Geometry: final body of the model. Coordinates: model frame, mm. A direction names the side the tool comes from. Give positions to 0.01 mm unless a question says otherwise; leave off trailing zeros. Write each loop counter-clockwise with the first axis right and the second up, starting at its lowest first coordinate (ties: lowest second). Pieces come first, ordered by that corner, then holes. Notation, with made-up numbers: M 85,58.5 L 93,58.5 A23 ccw 93,96.5 Z; hole C -12.5,-0.75 d3. An arc over 180 degrees is marked long. Use a Markdown table: item, result. Add a question column.
1) Section C-C on y = 42. Return the cut outline in (x, z), then the cut area to 3 significant figures.
2) Section B-B on z = 33. Return the cut outline in (x, y).
3) Set-up query: faces 1 (the cylindrical face through (4.83, 4.93, 18.22)), 2 (the flat face through (5, 43, 34)), 3 (the cylindrical face through (7.62, 3.78, 2)), 4 (the cylindrical face through (4.763, 77.521, 18.835)), 5 (the flat face through (7.5, 77, 34)). Return all of +Z, -Z, +X, -X, +Y, -Y with unobstructed straight access to the full face (end or side cutting, diameter ignored); none if empty.
4) Line query: line 1 (Z direction, x = 3.5, y = 4.5); line 2 (Y direction, x = 0.5, z = 27.5); line 3 (Z direction, x = 5, y = 2.5). Output: solid intervals per line, ascending.
5) Pin query (flat end, axial travel): pin 1 (4 mm diameter, centred on x = 11.5, z = 30, fed in from +Y); pin 2 (5 mm diameter, centred on x = 5, z = 21.5, fed in from +Y); pin 3 (2.5 mm diameter, centred on y = 77.5, z = 33, fed in from +X); pin 4 (2.5 mm diameter, centred on y = 41, z = 2, fed in from +X). Return the tip coordinate at first contact, or that it passes through.
6) Section D-D on z = 23. Return the cut outline in (x, y).
7) Draft query along X for faces 6 (the flat face through (7.5, 77, 4)), 7 (the cylindrical face through (4.733, 66.033, 36.028)), 8 (the flat face through (3, 76, 18)). Return one class per face: +X half, -X half, draft (parallel to the pull), parting line (faces both ways), or undercut.
8) Section A-A on y = 64. Return the cut outline in (x, z), then the cut area to 3 significant figures.
```python
from build123d import *

# Parameters (mm, degrees)
PAD_DEPTH       = 38
SKETCH001_R     = 2.05
POCKET_DEPTH    = 17.363189
SKETCH002_W     = 66
SKETCH002_H     = 31
POCKET001_DEPTH = 15.241
SKETCH003_R     = 2.05
POCKET002_DEPTH = 38.001
SKETCH004_W     = 3
SKETCH004_H     = 38
POCKET003_DEPTH = 2.5
POCKET004_DEPTH = 5
SKETCH006_R     = 0.8
POCKET005_DEPTH = 15


with BuildPart() as part:
    # Sketch → Pad (new body)
    with BuildSketch(Plane.XY):
        Polygon((15, 0), (0, 0), (0, 79), (10, 79), (10, 10), (15.24, 8), align=None)
    extrude(amount=PAD_DEPTH)

    # Sketch001 (on Face6 of Pad) → Pocket (cut, through all)
    with BuildSketch(Plane(origin=(14.986512, -0.449595, 0), x_dir=(0.029987, 0.99955, 0), z_dir=(0.99955, -0.029987, 0))):
        with Locations((4.451597, 34)):
            Circle(SKETCH001_R)
        with Locations((4.451597, 4)):
            Circle(SKETCH001_R)
    extrude(amount=-POCKET_DEPTH, mode=Mode.SUBTRACT)

    # Sketch002 (on Face3 of Pocket) → Pocket001 (cut, through all)
    with BuildSketch(Plane(origin=(0, 0, 0), x_dir=(0, -1, 0), z_dir=(-1, 0, 0))):
        with Locations((-43, 18.5)):
            Rectangle(SKETCH002_W, SKETCH002_H)
    extrude(amount=-POCKET001_DEPTH, mode=Mode.SUBTRACT)

    # Sketch003 (on Face5 of Pocket001) → Pocket002 (cut, through all)
    with BuildSketch(Plane.XY.offset(38)):
        with Locations((5, 64)):
            Circle(SKETCH003_R)
    extrude(amount=-POCKET002_DEPTH, mode=Mode.SUBTRACT)

    # Sketch004 (on Face14 of Pocket002) → Pocket003 (cut)
    with BuildSketch(Plane.YZ.offset(10)):
        with Locations((77.5, 19)):
            Rectangle(SKETCH004_W, SKETCH004_H)
    extrude(amount=-POCKET003_DEPTH, mode=Mode.SUBTRACT)

    # Sketch005 (on Face9 of Pocket003) → Pocket004 (cut)
    with BuildSketch(Plane(origin=(0, 79, 0), x_dir=(-1, 0, 0), z_dir=(0, 1, 0))):
        with BuildLine():
            ThreePointArc((-7.5, 7.624688), (-4.762126, 19), (-7.5, 30.375312))
            Line((-7.5, 7.624688), (-7.5, 30.375312))
        make_face()
    extrude(amount=-POCKET004_DEPTH, mode=Mode.SUBTRACT)

    # Sketch006 (on Face1 of Pocket004) → Pocket005 (cut)
    with BuildSketch(Plane.XZ):
        with Locations((5, 19)):
            Circle(SKETCH006_R)
    extrude(amount=-POCKET005_DEPTH, mode=Mode.SUBTRACT)


solid = part.part
```
Found:
| question | item | result |
|---|---|---|
| 1 | outline | M 0,0 L 10,0 L 10,3 L 0,3 Z; M 0,34 L 10,34 L 10,38 L 0,38 Z |
| 1 | area | 70.0 mm² |
| 2 | outline | M 0,0 L 15,0 L 15.07,2.21 L 0,2.66 Z; M 0,6.24 L 15.17,5.79 L 15.24,8 L 10,10 L 0,10 Z; M 0,76 L 7.5,76 L 7.5,79 L 0,79 Z |
| 3 | face 1 | -Y |
| 3 | face 2 | +X, -X |
| 3 | face 3 | none |
| 3 | face 4 | +X, +Y |
| 3 | face 5 | +Z, -Z, +X, +Y |
| 4 | line 1 | 0 to 1.96, 6.04 to 31.96, 36.04 to 38 |
| 4 | line 2 | 0 to 10, 76 to 79 |
| 4 | line 3 | 0 to 3.02, 4.98 to 18.2, 19.8 to 33.02, 34.98 to 38 |
| 5 | pin 1 | y = 10 |
| 5 | pin 2 | y = 79 |
| 5 | pin 3 | x = 7.5 |
| 5 | pin 4 | x = 10 |
| 6 | outline | M 0,0 L 15,0 L 15.24,8 L 10,10 L 0,10 Z; M 0,76 L 5.08,76 L 5.08,79 L 0,79 Z |
| 7 | face 6 | +X half |
| 7 | face 7 | undercut |
| 7 | face 8 | draft |
| 8 | outline | M 0,0 L 2.95,0 L 2.95,3 L 0,3 Z; M 0,34 L 2.95,34 L 2.95,38 L 0,38 Z; M 7.05,0 L 10,0 L 10,3 L 7.05,3 Z; M 7.05,34 L 10,34 L 10,38 L 7.05,38 Z |
| 8 | area | 41.3 mm² |
